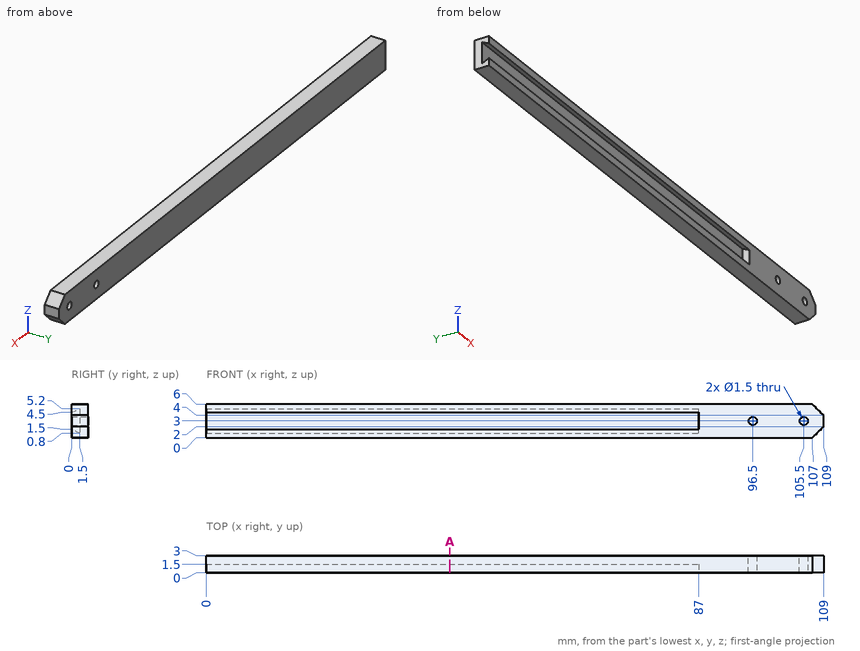
Print and shaded views of the part. All mm, measured from the part's lowest x, y and z. Round coordinates to 2 decimals unless told otherwise and drop trailing zeros. Loops run counter-clockwise (first coordinate to the right, second up) from the corner with the lowest first, then second, coordinate; pieces in that order, holes last. Notation, with made-up numbers: M 14,85 L 53,85 A21 ccw 53,124 Z; hole C 24,60 d1. An arc over 180 degrees is marked long. One line per question, with ' | ' between items.
1) Flat gauge pins, fed straight in: pin 1 (1.5 mm diameter, centred on y = 0.5, z = 3, fed in from -X); pin 2 (0.9 mm diameter, centred on x = 96.5, z = 3, fed in from -Y). Where does each tip first touch, or does it go through?
Solved:
pin 1: stops at x = 87 | pin 2: passes through
2) Band-saw the part on A-A (x = 43). Give the cut face in (y, z).
Solved:
outline: M 0,0 L 3,0 L 3,6 L 0,6 L 0,4.5 L 1.5,5.2 L 1.5,0.8 L 0,1.5 Z
3) Drill centre lines: line 1 along X through (y, z) = (1.55, 3); line 2 along Z through (x, y) = (96.5, 2.3); line 3 along X through (y, z) = (0.7, 3). Where is each one in solid material? Low to high.
Solved:
line 1: x = 0 to 95.75, 97.25 to 104.75, 106.25 to 109 | line 2: z = 0 to 2.25, 3.75 to 6 | line 3: x = 87 to 95.75, 97.25 to 104.75, 106.25 to 109
